For this review, take the finished solid that the model builds, in its own axes (mm). A direction names the side the tool comes from. Round coordinates to 2 decimals unless told otherwise and drop trailing zeros. Write each loop counter-clockwise with the first axis right and the second up, starting at its lowest first coordinate (ties: lowest second). Pieces come first, ordered by that corner, then holes.
from build123d import *

# Parameters (mm, degrees)
RETAINER_PLATE_START                       = 33.1
SKETCH1_W                                  = 7
SKETCH1_H                                  = 23
RETAINER_PLATE_DEPTH                       = 1.8
RETAINER_MOUNTING_SPACERS_START            = 34.9
SKETCH2_R                                  = 2
RETAINER_MOUNTING_SPACERS_DEPTH            = 0.1
RETAINER_CLEARANCE_HOLES_START             = 32
SKETCH3_R                                  = 1.7
SKETCH3_R_2                                = 1.1
RETAINER_CLEARANCE_HOLES_DEPTH             = 6
CLEAR_END_WALL_START                       = 33
SKETCH4_W                                  = 15
SKETCH4_H                                  = 6.3
CLEAR_END_WALL_DEPTH                       = 6
THUMB_MOUNT_EXTENSION_START                = 33.1
SKETCH5_W                                  = 7
SKETCH5_H                                  = 6
THUMB_MOUNT_EXTENSION_DEPTH                = 1.8
THUMB_MOUNT_PAD_START                      = 33.1
SKETCH6_R                                  = 5.75
THUMB_MOUNT_PAD_DEPTH                      = 1.8
THUMB_CLEARANCE_D7_START                   = 32.8
SKETCH7_R                                  = 3.5
THUMB_CLEARANCE_D7_DEPTH                   = 2.5
CLEAR_LEGACY_SPACER_FROM_THUMB_BOSS_START  = 34.9
SKETCH8_R                                  = 6.05
CLEAR_LEGACY_SPACER_FROM_THUMB_BOSS_DEPTH  = 2.3
FREE_SLIDING_BUTTON_LOWER_GUIDE_D3P6_START = 33
SKETCH9_R                                  = 1.8
FREE_SLIDING_BUTTON_LOWER_GUIDE_D3P6_DEPTH = 2
CUT_EXTRUDE2_START                         = 33
SKETCH10_R                                 = 1.8
CUT_EXTRUDE2_DEPTH                         = 2


with BuildPart() as part:
    # Sketch1 → Retainer_plate (new body)
    with BuildSketch(Plane.XY.offset(RETAINER_PLATE_START)):
        with Locations((-32.018684277, -38)):
            Rectangle(SKETCH1_W, SKETCH1_H)
    extrude(amount=RETAINER_PLATE_DEPTH)

    # Sketch2 → Retainer_mounting_spacers (add)
    with BuildSketch(Plane.XY.offset(RETAINER_MOUNTING_SPACERS_START)):
        with Locations(Location((-32.018684277, -47.5, 0), (0, 0, 270))):
            Circle(SKETCH2_R)
        with Locations(Location((-32.018684277, -28.5, 0), (0, 0, 90))):
            Circle(SKETCH2_R)
    extrude(amount=RETAINER_MOUNTING_SPACERS_DEPTH)

    # Sketch3 → Retainer_clearance_holes (cut)
    with BuildSketch(Plane.XY.offset(RETAINER_CLEARANCE_HOLES_START)):
        with Locations(Location((-32.018684277, -41.745416557, 0), (0, 0, 180))):
            Circle(SKETCH3_R)
        with Locations(Location((-32.018684277, -34.643402341, 0), (0, 0, 180))):
            Circle(SKETCH3_R)
        with Locations(Location((-32.018684277, -47.5, 0), (0, 0, 180))):
            Circle(SKETCH3_R_2)
        with Locations(Location((-32.018684277, -28.5, 0), (0, 0, 180))):
            Circle(SKETCH3_R_2)
    extrude(amount=RETAINER_CLEARANCE_HOLES_DEPTH, mode=Mode.SUBTRACT)

    # Sketch4 → Clear_end_wall (cut)
    with BuildSketch(Plane.XY.offset(CLEAR_END_WALL_START)):
        with Locations((-32.5, -51.85)):
            Rectangle(SKETCH4_W, SKETCH4_H)
    extrude(amount=CLEAR_END_WALL_DEPTH, mode=Mode.SUBTRACT)

    # Sketch5 → Thumb_mount_extension (add)
    with BuildSketch(Plane.XY.offset(THUMB_MOUNT_EXTENSION_START)):
        with Locations((-32.018684277, -25)):
            Rectangle(SKETCH5_W, SKETCH5_H)
    extrude(amount=THUMB_MOUNT_EXTENSION_DEPTH)

    # Sketch6 → Thumb_mount_pad (add)
    with BuildSketch(Plane.XY.offset(THUMB_MOUNT_PAD_START)):
        with Locations((-32.018684277, -22)):
            Circle(SKETCH6_R)
    extrude(amount=THUMB_MOUNT_PAD_DEPTH)

    # Sketch7 → Thumb_clearance_D7 (cut)
    with BuildSketch(Plane.XY.offset(THUMB_CLEARANCE_D7_START)):
        with Locations(Location((-32.018684277, -22, 0), (0, 0, 180))):
            Circle(SKETCH7_R)
    extrude(amount=THUMB_CLEARANCE_D7_DEPTH, mode=Mode.SUBTRACT)

    # Sketch8 → Clear_legacy_spacer_from_thumb_boss (cut)
    with BuildSketch(Plane.XY.offset(CLEAR_LEGACY_SPACER_FROM_THUMB_BOSS_START)):
        with Locations((-32.018684277, -22)):
            Circle(SKETCH8_R)
    extrude(amount=CLEAR_LEGACY_SPACER_FROM_THUMB_BOSS_DEPTH, mode=Mode.SUBTRACT)

    # Sketch9 → Free_sliding_button_lower_guide_D3p6 (cut)
    with BuildSketch(Plane.XY.offset(FREE_SLIDING_BUTTON_LOWER_GUIDE_D3P6_START)):
        with Locations(Location((-32.018684277, -41.745416557, 0), (0, 0, 180))):
            Circle(SKETCH9_R)
    extrude(amount=FREE_SLIDING_BUTTON_LOWER_GUIDE_D3P6_DEPTH, mode=Mode.SUBTRACT)

    # Sketch10 → Cut-Extrude2 (cut)
    with BuildSketch(Plane.XY.offset(CUT_EXTRUDE2_START)):
        with Locations(Location((-32.018684277, -34.643402341, 0), (0, 0, 180))):
            Circle(SKETCH10_R)
    extrude(amount=CUT_EXTRUDE2_DEPTH, mode=Mode.SUBTRACT)


solid = part.part
(1) For faces 1 (the face through (-32, -28, 34)), 2 (the face through (-35.519, -38, 34)), 3 (the face through (-32, -32, 33.1)), list the 3-axis set-ups (+Z, -Z, +X, -X, +Y, -Y) from which the entire face can be reached by the end or side of a thin tool; tool diameter is ignored.
Geometry check:
face 1: +Z, -Z
face 2: +Z, -Z, -X, -Y
face 3: -Z, +X, -X, +Y, -Y
(2) For pin 1 Ø0.5 at (y, z) = (-38.5, 34.5) entering from -X; pin 2 Ø0.9 at (y, z) = (-36.5, 34) entering from +X; pin 3 Ø1 at (x, z) = (-30, 33.5) entering from +Y, all flat-tipped, find the tip position at first contact; note any pin that passes through.
Geometry check:
pin 1: stops at x = -35.52
pin 2: stops at x = -28.52
pin 3: stops at y = -16.45
(3) We need section C-C, the plane y = -28.5. Give the boundary of the cut face in (x, z), and give its area (3 significant figures).
Geometry check:
outline: (-35.52, 33.1) - (-33.12, 33.1) - (-33.12, 35) - (-34.02, 35) - (-34.02, 34.9) - (-35.52, 34.9) - close; (-30.92, 33.1) - (-28.52, 33.1) - (-28.52, 34.9) - (-30.02, 34.9) - (-30.02, 35) - (-30.92, 35) - close
area: 8.82 mm2
(4) Mouldability with a two-part tool opening along X and no side actions: class faces 4 (the face through (-28.519, -38, 34)), 5 (the face through (-30.59, -40.65, 33.99)), 6 (the face through (-32, -46, 35)) as pulls with the +X half, pulls with the -X half, needs draft (parallel to the pull), parting line crosses it, or undercut.
Geometry check:
face 4: pulls with the +X half
face 5: undercut
face 6: needs draft
(5) We need section D-D, the plane y = -37.5. Give the boundary of the cut face in (x, z).
Geometry check:
outline: (-35.52, 33.1) - (-28.52, 33.1) - (-28.52, 34.9) - (-35.52, 34.9) - close
(6) For line 1 along Z through (x, y) = (-29.75, -26); line 2 along X through (y, z) = (-32, 34); line 3 along Y through (x, z) = (-33.75, 34.95), list the stretches that pass through material, from the lowest coordinate up.
Geometry check:
line 1: z = 33.1 to 34.9
line 2: x = -35.52 to -28.52
line 3: y = -48.5 to -46.5, -29.5 to -27.8
(7) We need section A-A, the plane y = -22. Give the boundary of the cut face in (x, z), and give its area (3 significant figures).
Geometry check:
outline: (-37.77, 33.1) - (-35.52, 33.1) - (-35.52, 34.9) - (-37.77, 34.9) - close; (-28.52, 33.1) - (-26.27, 33.1) - (-26.27, 34.9) - (-28.52, 34.9) - close
area: 8.10 mm2
(8) We need section B-B, the plane z = 34.55. Give the boundary of the cut face in (x, y), and give its area (3 significant figures).
Geometry check:
outline: (-35.52, -48.7) - (-28.52, -48.7) - (-28.52, -26.56) arc R5.75 ccw (long way) to (-35.52, -26.56) - close; hole circle Ø7 at (-32.02, -22); hole circle Ø3.6 at (-32.02, -41.75); hole circle Ø3.6 at (-32.02, -34.64); hole circle Ø2.2 at (-32.02, -47.5); hole (-33, -28) arc R1.1 ccw (long way) to (-31.04, -28) - close
area: 188 mm2
